```python
from build123d import *

# Parameters (mm, degrees)
SKETCH3_R          = 1.4
CUT_EXTRUDE1_DEPTH = 41.620192023
SKETCH5_R          = 1.5
CUT_EXTRUDE2_DEPTH = 40.230090492


with BuildPart() as part:
    # Sketch2 → Revolve1 (revolve)
    with BuildSketch(Plane(origin=(0, 0, 0), x_dir=(0, 0, -1), z_dir=(1, 0, 0)), mode=Mode.PRIVATE) as revolve1_sk:
        Polygon((10, 4), (10, 25), (7, 25), (7, 20), (-7, 20), (-7, 25), (-10, 25), (-10, 4), align=None)
    revolve(revolve1_sk.sketch.rotate(Axis((0, 0, 10), (0, 0, -1)), 90), axis=Axis((0, 0, 10), (0, 0, -1)))

    # Sketch3 → Cut-Extrude1 (cut, through all)
    with BuildSketch(Plane.XY.offset(10)):
        with Locations((0, 10)):
            Circle(SKETCH3_R)
        with Locations((8.660254038, 5)):
            Circle(SKETCH3_R)
        with Locations((8.660254038, -5)):
            Circle(SKETCH3_R)
        with Locations((0, -10)):
            Circle(SKETCH3_R)
        with Locations((-8.660254038, -5)):
            Circle(SKETCH3_R)
        with Locations((-8.660254038, 5)):
            Circle(SKETCH3_R)
    extrude(amount=-CUT_EXTRUDE1_DEPTH, mode=Mode.SUBTRACT)

    # Sketch5 → Cut-Extrude2 (cut, through all)
    with BuildSketch(Plane(origin=(0, 0, 7), x_dir=(-1, 0, 0), z_dir=(0, 0, -1))):
        with Locations((-4, 22)):
            Circle(SKETCH5_R)
        with Locations((4, 22)):
            Circle(SKETCH5_R)
    extrude(amount=-CUT_EXTRUDE2_DEPTH, mode=Mode.SUBTRACT)


solid = part.part
```
Build history of the part. All positions in model axes, mm. A direction names the side the tool comes from. Round coordinates to 2 decimals unless told otherwise and drop trailing zeros. Order: outer loops, then holes, each group sorted by start corner. A loop starts at its lowest first (then second) coordinate and runs counter-clockwise, first axis right, second up. Notation, with made-up numbers: (69, 71.5) -> (92, 71.5) arc R19 cw to (92, 75.5) -> close; hole circle Ø2 at (30.25, 68). An arc over 180 degrees is marked (long way). Answer in a Markdown table with one row per item.
1) Mould opens along X. For faces 1 (the cylindrical face through (-4.806, 23.265, 8.479)), 2 (the cylindrical face through (23.846, -7.509, -8.479)), 3 (the flat face through (-5, 0, -10)) say: released by +X, released by -X, zero draft, split by the parting line, or undercut.
Values:
| item | result |
|---|---|
| face 1 | undercut |
| face 2 | split by the parting line |
| face 3 | zero draft |
2) Band-saw the part on B-B on x = 0. Give the cut face in (y, z).
Values:
| item | result |
|---|---|
| outline | (-25, -10) -> (-11.4, -10) -> (-11.4, 10) -> (-25, 10) -> (-25, 7) -> (-20, 7) -> (-20, -7) -> (-25, -7) -> close; (-8.6, -10) -> (-4, -10) -> (-4, 10) -> (-8.6, 10) -> close; (4, -10) -> (8.6, -10) -> (8.6, 10) -> (4, 10) -> close; (11.4, -10) -> (25, -10) -> (25, -7) -> (20, -7) -> (20, 7) -> (25, 7) -> (25, 10) -> (11.4, 10) -> close |
3) Band-saw the part on A-A on z = -8.25. Give the cut face in (x, y).
Values:
| item | result |
|---|---|
| outline | circle Ø50 at (0, 0); hole circle Ø2.8 at (-8.66, -5); hole circle Ø2.8 at (-8.66, 5); hole circle Ø8 at (0, 0); hole circle Ø2.8 at (0, -10); hole circle Ø2.8 at (0, 10); hole circle Ø2.8 at (8.66, -5); hole circle Ø2.8 at (8.66, 5) |
4) Pin check, flat tips, straight feed: P1, Ø5, axis at x = 10.5, z = 8, coming from the +Y side; P2, Ø1.7, axis at x = 0, y = -10, coming from the -Z side; P3, Ø2, axis at x = -2.5, z = 3, coming from the -Y side; P4, Ø12, axis at x = 5, z = -5, coming from the +Y side. Stop position of each tip, or through.
Values:
| item | result |
|---|---|
| P1 | y = 23.69 |
| P2 | through |
| P3 | y = -19.94 |
| P4 | y = 25 |
5) Band-saw the part on D-D on z = 8. Give the number of separate pieces and of enclosed holes in the cut face, and give its area (3 significant figures).
Values:
| item | result |
|---|---|
| separate pieces | 1 |
| enclosed holes | 9 |
| area | 1,860 mm2 |
6) Wall check: L1, parallel to Z at x = 7, y = -21.5; L2, parallel to Y at x = -8, z = -0.5; L3, parallel to X at y = 10.5, z = -8. Give the ranges that are in metal, low to high.
Values:
| item | result |
|---|---|
| L1 | -10 to -7, 7 to 10 |
| L2 | -18.33 to -6.23, -3.77 to 3.77, 6.23 to 18.33 |
| L3 | -22.69 to -1.31, 1.31 to 22.69 |
7) Which spindle directions (+Z, -Z, +X, -X, +Y, -Y) get a long thin tool onto all of the face, cutting with end or side? Do faces 4 (the cylindrical face through (-19.98, -0.88, 0.1)), 5 (the cylindrical face through (4.195, 23.487, 8.479)), 6 (the cylindrical face through (-7.37, -5.54, 0.14)). Say none if no direction does.
Values:
| item | result |
|---|---|
| face 4 | none |
| face 5 | +Z |
| face 6 | +Z, -Z |
8) Band-saw the part on C-C on y = 0. Give the cut face in (x, z), and give its area (3 significant figures).
Values:
| item | result |
|---|---|
| outline | (-25, -10) -> (-4, -10) -> (-4, 10) -> (-25, 10) -> (-25, 7) -> (-20, 7) -> (-20, -7) -> (-25, -7) -> close; (4, -10) -> (25, -10) -> (25, -7) -> (20, -7) -> (20, 7) -> (25, 7) -> (25, 10) -> (4, 10) -> close |
| area | 700 mm2 |
